The listing builds one solid part. Answer for the finished solid, in the listing's coordinates (mm). Face numbers are marked on the shaded views. A direction names the side the tool comes from. Give positions to 0.01 mm unless a question says otherwise; leave off trailing zeros. Order: outer loops, then holes, each group sorted by start corner. A loop starts at its lowest first (then second) coordinate and runs counter-clockwise, first axis right, second up. Notation, with made-up numbers: M 63.25,-21 L 90.25,-21 A6 ccw 90.25,-16 Z; hole C 5.5,33 d4. An arc over 180 degrees is marked long. Answer as a JSON object with one key per item and string values. Group by question number.
```python
from build123d import *

# Parameters (mm, degrees)
SKETCH1_W           = 15.24
SKETCH1_H           = 6.096
BOSS_EXTRUDE1_DEPTH = 2.54
SHELL1_T            = -0.635
FILLET1_R           = 0.635
SKETCH2_R           = 1.5875
BOSS_EXTRUDE2_DEPTH = 1.905
BOSS_EXTRUDE3_DEPTH = 0.00254


with BuildPart() as part:
    # Sketch1 → Boss-Extrude1 (new body)
    with BuildSketch(Plane(origin=(0, 0, 0), x_dir=(1, 0, 0), z_dir=(0, 1, 0))):
        with Locations((7.62, 3.048)):
            Rectangle(SKETCH1_W, SKETCH1_H)
    extrude(amount=BOSS_EXTRUDE1_DEPTH)

    # Shell1
    shell1_openings = [part.faces().sort_by_distance(p)[0] for p in [
        (7.62, 0, -3.048),
    ]]
    offset(amount=SHELL1_T, openings=shell1_openings, kind=Kind.INTERSECTION)

    # Fillet1
    fillet1_edges = [part.edges().sort_by_distance(p)[0] for p in [
        (0, 1.27, 0),
        (15.24, 1.27, 0),
        (15.24, 1.27, -6.096),
        (0, 1.27, -6.096),
    ]]
    fillet(fillet1_edges, radius=FILLET1_R)

    # Sketch2 → Boss-Extrude2 (add)
    with BuildSketch(Plane.XZ.offset(-1.905)):
        with Locations(Location((7.62, -3.048, 0), (0, 0, 270))):
            Circle(SKETCH2_R)
    extrude(amount=BOSS_EXTRUDE2_DEPTH)

    # Sketch3 → Boss-Extrude3 (add)
    with BuildSketch(Plane(origin=(0, 2.54, 0), x_dir=(1, 0, 0), z_dir=(0, 1, 0))):
        Polygon((7.251008013, 4.445), (7.669507612, 4.445), (8.558660256, 2.084102564), (8.042213942, 2.084102564), (7.459621795, 3.630897436), (6.87639363, 2.084102564), (6.360583333, 2.084102564), align=None)
    extrude(amount=BOSS_EXTRUDE3_DEPTH)


solid = part.part
```
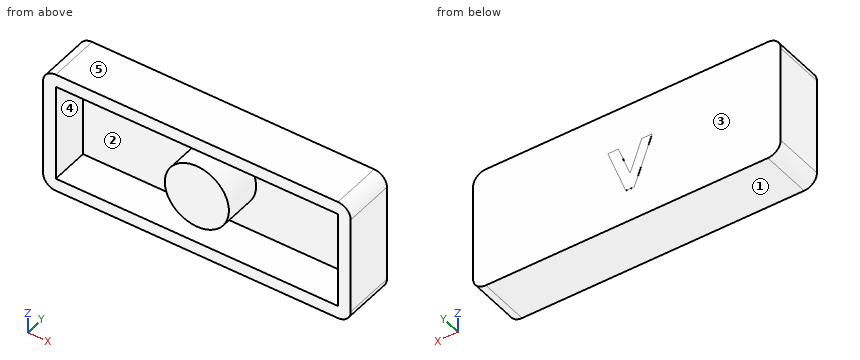
Item 1: Section C-C (z = -5.25) is taken. Determine the outline of the cut face in (x, y) (3 decimals).
Item 2: Determine the mould class of the marked faces 3, 4 and 5 for opening direction Z: released by +Z, released by -Z, zero draft, split by the parting line, or undercut.
Item 3: Section B-B (x = 13) is taken. Determine the outline of the cut face in (y, z) (3 decimals), and give its area (3 significant figures).
Item 4: A flat-ended cylindrical pin translates along its axis: P1, Ø2.5, axis at x = 11, z = -3, coming from the -Y side (3 decimals). Find the tip coordinate at first contact, or state that the pin passes through.
Item 5: Consider probe 1 along X at (y, z) = (0.35, -3) (3 decimals); probe 2 along Z at (x, y) = (14.5, 1.7) (3 decimals); probe 3 along X at (y, z) = (0.85, -4.5) (3 decimals). Determine where each line is inside the solid, lowest interval first. Write a range as from..to.
Item 6: A tool of negligible diameter and unlimited length cuts with its end or side. For the marked faces 1 and 2, from which of +Z, -Z, +X, -X, +Y, -Y can it reach the whole face along a straight path? Write none if from no direction.
Item 7: Section A-A (y = 1.5) is taken. Determine the outline of the cut face in (x, z) (1 decimal), and give its area (3 significant figures).
Values found:
{
 "1": {"outline": "M 0,0 L 0.635,0 L 0.635,1.905 L 14.605,1.905 L 14.605,0 L 15.24,0 L 15.24,2.54 L 0,2.54 Z"},
 "2": {"face 3": "zero draft", "face 4": "undercut", "face 5": "released by +Z"},
 "3": {"outline": "M 0,-6.096 L 2.54,-6.096 L 2.54,0 L 0,0 L 0,-0.635 L 1.905,-0.635 L 1.905,-5.461 L 0,-5.461 Z", "area": "6.29 mm^2"},
 "4": {"P1": "stops at y = 1.905"},
 "5": {"probe 1": "x = 0..0.635, 6.033..9.207, 14.605..15.24", "probe 2": "z = -6.096..-5.461, -0.635..0", "probe 3": "x = 0..0.635, 6.978..8.262, 14.605..15.24"},
 "6": {"face 1": "-Z, +X, -X, +Y, -Y", "face 2": "-Y"},
 "7": {"outline": "M 0,-5.5 A0.6 ccw 0.6,-6.1 L 14.6,-6.1 A0.6 ccw 15.2,-5.5 L 15.2,-0.6 A0.6 ccw 14.6,0 L 0.6,0 A0.6 ccw 0,-0.6 Z; C 7.6,-3 d3.2; hole M 0.6,-5.5 L 14.6,-5.5 L 14.6,-0.6 L 0.6,-0.6 Z", "area": "33.1 mm^2"}
}
